Part print with two shaded views. Sizes in mm from the minimum x, y, z corner. A direction names the side the tool comes from. Coordinates: 2 decimals unless noted, no trailing zeros. Loops run counter-clockwise (first coordinate to the right, second up) from the corner with the lowest first, then second, coordinate; pieces in that order, holes last.
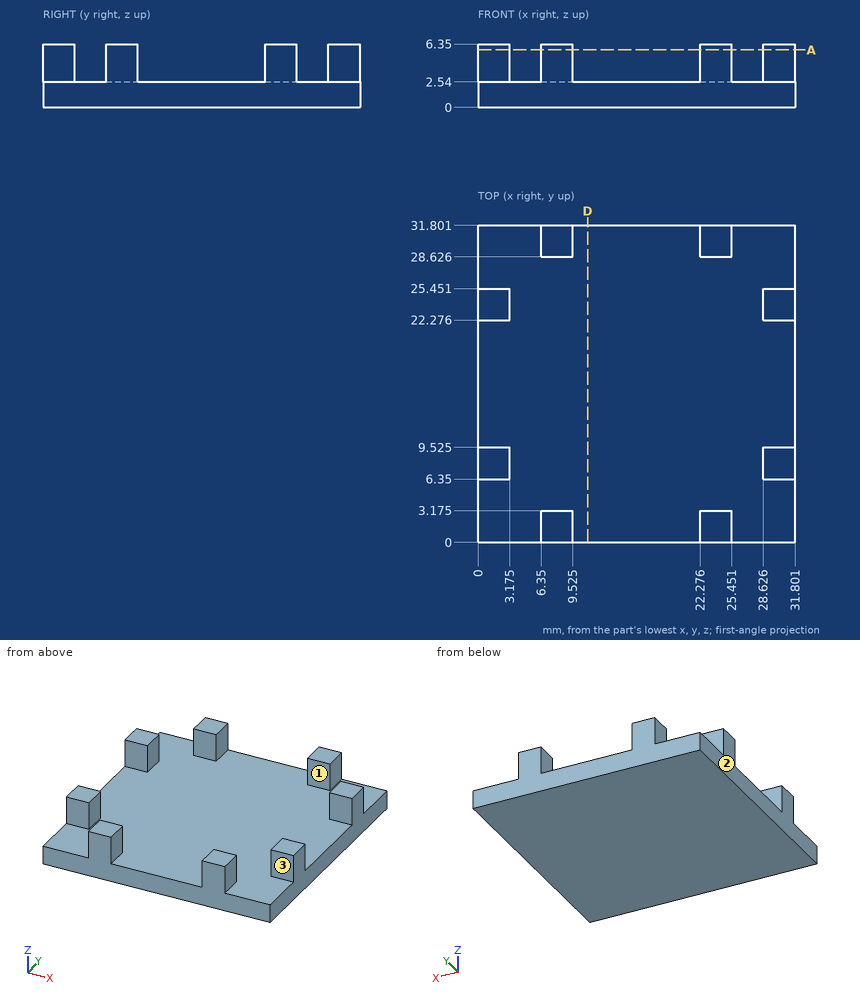
Q1. Drill centre lines: line 1 (Y direction, x = 25, z = 5) (1 decimal); line 2 (Z direction, x = 15.5, y = 25). Where is each one in solid material? Low to high.
Answers:
line 1: y = 0 to 3.2, 28.6 to 31.8
line 2: z = 0 to 2.54
Q2. Flat gauge pins, fed straight in: P1, Ø2.5, axis at y = 29.5, z = 5, coming from the +X side; P2, Ø3.5, axis at x = 2, z = 5, coming from the -Y side; P3, Ø1, axis at y = 2, z = 4.5, coming from the -X side. Where does each tip first touch, or does it go through?
Answers:
P1: stops at x = 25.45
P2: stops at y = 6.35
P3: stops at x = 6.35
Q3. Slice it at D-D (x = 11). List the corners of the cut face in (y, z).
Answers:
outline: (0, 0) - (31.8, 0) - (31.8, 2.54) - (0, 2.54) - close
Q4. Slice it at A-A (z = 5.75). Count the separate pieces of the cut face and the enclosed holes in it.
Answers:
separate pieces: 8
enclosed holes: 0
Q5. Which spindle directions (+Z, -Z, +X, -X, +Y, -Y) get a long thin tool onto all of the face, cutting with end or side? Do the marked faces 1, 2 and 3. Say none if no direction does.
Answers:
face 1: +Z, +X, -X
face 2: +Z, -Z, -X, +Y, -Y
face 3: +Z, +X, -X, -Y
